Verification items for the finished model (mm, model axes). Give positions to 0.01 mm unless a question says otherwise; leave off trailing zeros. Loops run counter-clockwise (first coordinate to the right, second up) from the corner with the lowest first, then second, coordinate; pieces in that order, holes last. Notation, with made-up numbers: M 84,37.25 L 127,37.25 A9 cw 127,43.25 Z; hole C 78.5,68 d11. An arc over 180 degrees is marked long. Use a Markdown table: item, result.
Autodesk Inventor part; units mm, degrees
ref_plane "YZ Plane" through (0, 0, 0) normal (1, 0, 0) x (0, 1, 0)
ref_plane "XZ Plane" through (0, 0, 0) normal (0, 1, 0) x (-1, 0, 0)
ref_plane "XY Plane" through (0, 0, 0) normal (0, 0, 1) x (1, 0, 0)
sketch "Sketch1" plane through (0, 0, 0) normal (0, 0, 1) x (1, 0, 0)
  line L0 (263.525, -215.9) -> (-263.525, -215.9)
  line L1 (-263.525, -215.9) -> (-263.525, 215.9)
  line L2 (-263.525, 215.9) -> (263.525, 215.9)
  line L3 (263.525, 215.9) -> (263.525, -215.9)
  line L4 (263.525, -215.9) -> (-263.525, 215.9) construction
  line L5 (-263.525, -215.9) -> (263.525, 215.9) construction
  point P0 (0, 0)
  dimension "d0" = 527.05
  dimension "d1" = 431.8
extrude "Extrusion1" add sketch "Sketch1" along normal blind 431.8
sketch "Sketch2" plane through (-263.525, 215.9, 0) normal (0, 1, 0) x (1, 0, 0)
  circle A0 centre (88.646, -61.722) radius 26.67
  point P0 (263.525, 0)
  dimension "d4" = 53.34
extrude "Extrusion2" cut sketch "Sketch2" against normal blind 431.8
properties part number "Sump Baffle Tub"
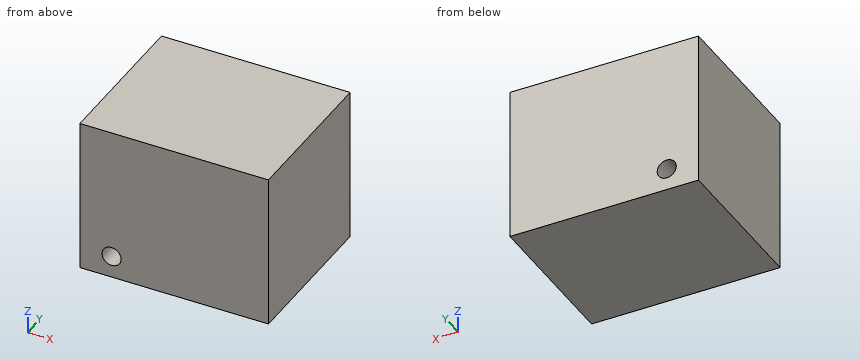
(1) Cross-section at A-A on x = -173. Record the cut outline in (y, z).
Results below:
| item | result |
|---|---|
| outline | M -215.9,0 L 215.9,0 L 215.9,35.12 L -215.9,35.12 Z; M -215.9,88.33 L 215.9,88.33 L 215.9,431.8 L -215.9,431.8 Z |
(2) Gauge pin test, flat end, axial feed: P1, Ø5, axis at x = -149, y = 114, coming from the -Z side. Record the tip position at first contact, or that the pin passes through.
Results below:
| item | result |
|---|---|
| P1 | z = 0 |
(3) Material ranges on line 1 (X direction, y = -167.5, z = 44) (3 decimals); line 2 (Z direction, x = -185.5, y = -127.5); line 3 (Z direction, x = -161, y = -10), recorded low to high.
Results below:
| item | result |
|---|---|
| line 1 | -263.525 to -194.809, -154.949 to 263.525 |
| line 2 | 0 to 37.26, 86.19 to 431.8 |
| line 3 | 0 to 38.95, 84.5 to 431.8 |
